Check sheet for the modelled part. Datum: model origin and axes. Units: mm. Round coordinates to 2 decimals unless told otherwise and drop trailing zeros. Order: outer loops, then holes, each group sorted by start corner. A loop starts at its lowest first (then second) coordinate and runs counter-clockwise, first axis right, second up.
```python
from build123d import *

# Parameters (mm, degrees)
SKETCH2_R           = 29.5
BOSS_EXTRUDE1_DEPTH = 5
SKETCH3_R           = 22.5
BOSS_EXTRUDE2_DEPTH = 100
CUT_EXTRUDE1_DEPTH  = 181


with BuildPart() as part:
    # Sketch2 → Boss-Extrude1 (new body)
    with BuildSketch(Plane(origin=(0, 0, 0), x_dir=(1, 0, 0), z_dir=(0, 1, 0))):
        with Locations(Location((0, 0, 0), (0, 0, 270))):
            Circle(SKETCH2_R)
    extrude(amount=BOSS_EXTRUDE1_DEPTH)

    # Sketch3 → Boss-Extrude2 (add)
    with BuildSketch(Plane.XZ):
        with Locations(Location((0, 0, 0), (0, 0, 270))):
            Circle(SKETCH3_R)
    extrude(amount=BOSS_EXTRUDE2_DEPTH)

    # Sketch4 → Cut-Extrude1 (cut)
    with BuildSketch(Plane(origin=(-63.996216882, 0, 59.671888061), x_dir=(0.6819644349807488, 0, 0.7313853357987076), z_dir=(-0.7313853357987076, 0, 0.6819644349807488))):
        with BuildLine():
            Line((-29.125423753, -34.169486826), (-29.125423753, -106.993301149))
            Line((-29.125423753, -106.993301149), (28.333748465, -106.993301149))
            Line((28.333748465, -106.993301149), (28.333748465, -22.496404242))
            add(Edge.make_bspline(
                [(-29.125423753, -34.169486826), (-19.027495219, -34.227173533), (-4.480834303, -34.028222863), (14.926714819, -29.772095296), (24.25688535, -26.283529721), (28.333748465, -22.496404242)],
                knots=[0, 0, 0, 0, 0.508723689, 0.724602868, 1, 1, 1, 1], degree=3))
        make_face()
    extrude(amount=-CUT_EXTRUDE1_DEPTH, mode=Mode.SUBTRACT)


solid = part.part
```
Item 1: Sectioned sample at A-A (y = 1). Record the cut outline in (x, z).
Answer:
outline: circle Ø59 at (0, 0)
Item 2: Sectioned sample at B-B (y = -15). Record the cut outline in (x, z).
Answer:
outline: circle Ø45 at (0, 0)
Item 3: Go/stop test with flat-tipped pins: P1, Ø5, axis at x = -19, y = -7.5, coming from the +Z side; P2, Ø5, axis at x = 4.5, y = -13.5, coming from the -Z side; P3, Ø1, axis at y = -21, z = -21, coming from the -X side. Record where each tip stops, or that it passes through.
Answer:
P1: stops at z = 15.3
P2: stops at z = -22.41
P3: stops at x = -9.27
Item 4: Scan lines: line 1 along Y through (x, z) = (-12, 21.5); line 2 along Z through (x, y) = (19, -8.5); line 3 along Y through (x, z) = (13.5, -14). Record each from-to range of solid material in increasing order.
Answer:
line 1: y = 0 to 5
line 2: z = -12.05 to 12.05
line 3: y = -32.85 to 5
Item 5: Release check for a two-part mould opening along Z. For faces 1 (the flat face through (0, 5, 0)), 2 (the cylindrical face through (8.86, 2.46, 28.14)) record: released by +Z, released by -Z, zero draft, split by the parting line, or undercut.
Answer:
face 1: zero draft
face 2: split by the parting line
